The model under review builds one solid part; all positions refer to its coordinate system, in mm. Round coordinates to 2 decimals unless told otherwise and drop trailing zeros. Order: outer loops, then holes, each group sorted by start corner. A loop starts at its lowest first (then second) coordinate and runs counter-clockwise, first axis right, second up. Notation, with made-up numbers: (31, -7.5) - (72, -7.5) arc R26 ccw to (72, 10.5) - close; hole circle Ø1 at (25.25, 68.5). An arc over 180 degrees is marked (long way). One line per question, with ' | ' between items. Start each with the question number.
Item 1: For L1, parallel to Y at x = -48.5, z = -21.5; L2, parallel to Y at x = -7.5, z = 14; L3, parallel to Y at x = -16, z = 23.5, list the stretches that pass through material, from the lowest coordinate up. Write a range as [from, to].
Item 2: Draft analysis for pull direction Y (two halves, no side actions). For faces 1 (the face through (-28, 5, -30)), 2 (the face through (-38.65, 5.08, 0.42)), 3 (the face through (-28, 7.302, 0)), state which applies: +Y half, -Y half, draft (parallel to the pull), parting line (faces both ways), or undercut.
Item 3: Insertion check: pin 1 Ø4 at (x, y) = (3.81, 1.905) entering from +Z. The pin has a flat end and moves straight along its axis. Give the tip position at first contact, or say it passes through.
Item 4: Add section B-B on y = 3.75. State how many separate pieces and enclosed holes the cut face has, and give its area (3 significant figures).
Item 5: Add section A-A on x = 3.81. State the section outline as (y, z) points.
from build123d import *

# Parameters (mm, degrees)
BOSS_EXTRUDE1_DEPTH    = 30
FILLET1_R              = 0.254
LPATTERN1_COUNT        = 10
LPATTERN1_PITCH        = 7.0612
FILLET1_OF_LPATTERN1_R = 0.254
SKETCH4_W              = 71.1708
SKETCH4_H              = 60
BOSS_EXTRUDE2_DEPTH    = 1.5875


with BuildPart() as part:
    # Sketch1 → Boss-Extrude1 (new, symmetric)
    with BuildSketch(Plane.XY):
        with BuildLine():
            Line((0, 0), (1.27, 0))
            ThreePointArc((1.27, 0), (3.81, 5.08), (6.35, 0))
            Line((6.35, 0), (7.62, 0))
            Line((7.62, 0), (7.62, 5.715))
            Line((7.62, 5.715), (0, 5.715))
            Line((0, 5.715), (0, 0))
        make_face()
    boss_extrude1 = extrude(amount=BOSS_EXTRUDE1_DEPTH, both=True)

    # Fillet1
    fillet1_edges = [part.edges().sort_by_distance(p)[0] for p in [
        (6.35, 0, 0),
        (1.27, 0, 0),
    ]]
    fillet(fillet1_edges, radius=FILLET1_R)

    # LPattern1: Boss-Extrude1 ×10
    with Locations(*[(-i * LPATTERN1_PITCH, 0, 0) for i in range(1, LPATTERN1_COUNT)]):
        add(boss_extrude1)

    # Fillet1 of LPattern1
    fillet1_of_lpattern1_edges = [part.edges().sort_by_distance(p)[0] for p in [
        (-0.7112, 0, 0),
        (-5.7912, 0, 0),
        (-7.7724, 0, 0),
        (-12.8524, 0, 0),
        (-14.8336, 0, 0),
        (-19.9136, 0, 0),
        (-21.8948, 0, 0),
        (-26.9748, 0, 0),
        (-28.956, 0, 0),
        (-34.036, 0, 0),
        (-36.0172, 0, 0),
        (-41.0972, 0, 0),
        (-43.0784, 0, 0),
        (-48.1584, 0, 0),
        (-50.1396, 0, 0),
        (-55.2196, 0, 0),
        (-57.2008, 0, 0),
        (-62.2808, 0, 0),
    ]]
    fillet(fillet1_of_lpattern1_edges, radius=FILLET1_OF_LPATTERN1_R)

    # Sketch4 → Boss-Extrude2 (add)
    with BuildSketch(Plane(origin=(0, 5.715, 0), x_dir=(1, 0, 0), z_dir=(0, 1, 0))):
        with Locations((-27.9654, 0)):
            Rectangle(SKETCH4_W, SKETCH4_H)
    extrude(amount=BOSS_EXTRUDE2_DEPTH)


solid = part.part
Determined:
1) L1: [0.03, 0.57], [3.24, 7.3] | L2: [0.09, 0.43], [3.38, 7.3] | L3: [4.77, 7.3]
2) face 1: draft | face 2: undercut | face 3: +Y half
3) pin 1: through
4) separate pieces: 11 | enclosed holes: 0 | area: 1,170 mm2
5) outline: (5.08, -30) - (7.3, -30) - (7.3, 30) - (5.08, 30) - close
